from build123d import *

# Parameters (mm, degrees)
SKETCH1_R      = 1.6
SKETCH1_R_2    = 1.3
EXTRUDE1_DEPTH = 3


with BuildPart() as part:
    # Sketch1 → Extrude1 (new body)
    with BuildSketch(Plane.XY):
        Polygon((-70, 34.003545781), (0, 34.003545781), (10, 24.003545781), (10, -64.753959847), (25, -79.753959847), (25, -169.753959847), (15, -179.753959847), (0, -179.753959847), (-70, -179.753959847), (-80, -169.753959847), (-80, 24.003545781), align=None)
        with Locations((-75, 2.893545781)):
            Circle(SKETCH1_R, mode=Mode.SUBTRACT)
        with Locations((-18.946632771, 2.893545781)):
            Circle(SKETCH1_R, mode=Mode.SUBTRACT)
        with Locations((-75, -142.403959847)):
            Circle(SKETCH1_R, mode=Mode.SUBTRACT)
        with Locations((-18.893164364, -142.403959847)):
            Circle(SKETCH1_R, mode=Mode.SUBTRACT)
        with Locations((4, 14.243545781)):
            Circle(SKETCH1_R_2, mode=Mode.SUBTRACT)
        with Locations((-50.5, 28.003545781)):
            Circle(SKETCH1_R_2, mode=Mode.SUBTRACT)
    extrude(amount=EXTRUDE1_DEPTH)


solid = part.part
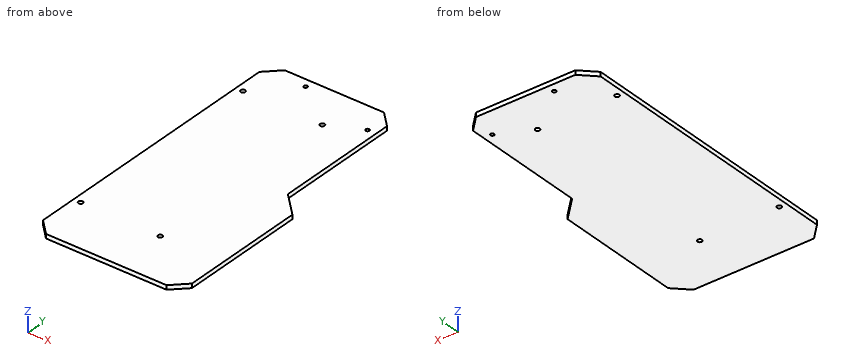
Here's how the part is built. I have some questions about the finished solid (model axes, mm). Coordinates: 2 decimals unless noted, no trailing zeros. Order: outer loops, then holes, each group sorted by start corner. A loop starts at its lowest first (then second) coordinate and runs counter-clockwise, first axis right, second up. Notation, with made-up numbers: (-5, -5) -> (14, -5) arc R16 cw to (14, 11) -> close; hole circle Ø10 at (-4.5, 73.25). An arc over 180 degrees is marked (long way). Answer in a Markdown table with one row per item.
(1) I want a section at A-A on z = 0.7. List the corners of the cut face in (x, y) for me, then the cut area to 3 significant figures.
Answer key:
| item | result |
|---|---|
| outline | (-80, -169.75) -> (-70, -179.75) -> (15, -179.75) -> (25, -169.75) -> (25, -79.75) -> (10, -64.75) -> (10, 24) -> (0, 34) -> (-70, 34) -> (-80, 24) -> close; hole circle Ø3.2 at (-75, -142.4); hole circle Ø3.2 at (-75, 2.89); hole circle Ø2.6 at (-50.5, 28); hole circle Ø3.2 at (-18.95, 2.89); hole circle Ø3.2 at (-18.89, -142.4); hole circle Ø2.6 at (4, 14.24) |
| area | 20,600 mm^2 |
(2) I want a section at B-B on y = -25.5. List the corners of the cut face in (x, z) for me, then the cut area to 3 significant figures.
Answer key:
| item | result |
|---|---|
| outline | (-80, 0) -> (10, 0) -> (10, 3) -> (-80, 3) -> close |
| area | 270 mm^2 |
(3) Will these pins go through, and if not, where does the flat tip stop? pin 1 Ø3 at (x, y) = (-18.89, -142.4) entering from -Z; pin 2 Ø1.5 at (y, z) = (-29, 1.5) entering from +X.
Answer key:
| item | result |
|---|---|
| pin 1 | through |
| pin 2 | x = 10 |
(4) Please list where these lines run through material, in increasing order: probe 1 along Y at (x, z) = (-75, 1.2); probe 2 along X at (y, z) = (3.5, 0.85); probe 3 along Y at (x, z) = (-50.5, 1.1).
Answer key:
| item | result |
|---|---|
| probe 1 | -174.75 to -144, -140.8 to 1.29, 4.49 to 29 |
| probe 2 | -80 to -76.48, -73.52 to -20.43, -17.47 to 10 |
| probe 3 | -179.75 to 26.7, 29.3 to 34 |
(5) I want a section at C-C on x = 12.5. List the corners of the cut face in (y, z) for me.
Answer key:
| item | result |
|---|---|
| outline | (-179.75, 0) -> (-67.25, 0) -> (-67.25, 3) -> (-179.75, 3) -> close |
